from build123d import *

# Parameters (mm, degrees)
BOSS_EXTRUDE1_DEPTH = 2.25
BOSS_EXTRUDE2_DEPTH = 2
CHAMFER1_SIZE       = 2
SKETCH2_R           = 2.1
CUT_EXTRUDE3_DEPTH  = 4.25
BOSS_EXTRUDE3_REACH = 165.691
SKETCH4_W           = 30.977136558
SKETCH4_H           = 2.25


with BuildPart() as part:
    # Sketch1 → Boss-Extrude1 (new body)
    with BuildSketch(Plane(origin=(0, 30, 0), x_dir=(1, 0, 0), z_dir=(0, 1, 0))):
        with BuildLine():
            Line((16.150801753, 24.75), (-16.150801753, 24.75))
            ThreePointArc((-16.150801753, 24.75), (-28.096079542, 23.126243037), (-39.174486808, 18.372808426))
            Line((-39.174486808, 18.372808426), (-74.75, -2.97249949))
            Line((-74.75, -2.97249949), (-74.75, -31.794317372))
            add(Edge.make_bspline(
                [(-74.75, -31.794317372), (-74.75, -34.854957393), (-74.617964132, -37.896617098), (-74.092634279, -43.942380332), (-73.699378084, -46.946489294), (-72.640258958, -52.915519667), (-71.97459072, -55.880469065), (-70.750169489, -60.295417047), (-70.303298869, -61.763844969), (-69.338133577, -64.660739638), (-68.819099262, -66.092346674), (-67.147343369, -70.334199296), (-65.881052999, -73.091977263), (-63.717003155, -77.10639512), (-62.951317542, -78.424051782), (-61.728649984, -80.366285253), (-61.307989229, -81.009022825), (-60.443810311, -82.277119387), (-60.001044485, -82.901462706), (-57.731833326, -85.972836279), (-55.741550679, -88.270936188), (-52.431333352, -91.422844474), (-51.271504838, -92.425348837), (-48.832250491, -94.308303199), (-47.564474204, -95.179986516), (-46.242530751, -95.973152587)],
                knots=[0, 0, 0, 0, 0.125, 0.125, 0.25, 0.25, 0.375, 0.375, 0.4375, 0.4375, 0.5, 0.5, 0.625, 0.625, 0.6875, 0.6875, 0.71875, 0.71875, 0.75, 0.75, 0.875, 0.875, 0.9375, 0.9375, 1, 1, 1, 1], degree=3))
            Line((-46.242530751, -95.973152587), (-31.73109903, -104.68001162))
            add(Edge.make_bspline(
                [(-31.73109903, -104.68001162), (-29.275377335, -106.153444637), (-26.68234242, -107.275661914), (-22.580548307, -108.4161221), (-21.170611667, -108.705239228), (-18.343968581, -109.085294073), (-16.920969223, -109.178932188), (-15.488568279, -109.178932188)],
                knots=[0, 0, 0, 0, 0.5, 0.5, 0.75, 0.75, 1, 1, 1, 1], degree=3))
            Line((-15.488568279, -109.178932188), (15.488568279, -109.178932188))
            add(Edge.make_bspline(
                [(15.488568279, -109.178932188), (18.352407294, -109.178932188), (21.153292414, -108.807120107), (25.257313775, -107.674700988), (26.615074004, -107.197210462), (29.234437058, -106.068808934), (30.502825354, -105.416975826), (31.73109903, -104.68001162)],
                knots=[0, 0, 0, 0, 0.5, 0.5, 0.75, 0.75, 1, 1, 1, 1], degree=3))
            Line((31.73109903, -104.68001162), (46.242530751, -95.973152587))
            add(Edge.make_bspline(
                [(46.242530751, -95.973152587), (47.567869145, -95.177949551), (48.829466075, -94.309558847), (51.243712939, -92.447684976), (52.396262721, -91.454086815), (54.604509349, -89.355684378), (55.660153085, -88.25081912), (57.177112794, -86.517159458), (57.67228307, -85.925631056), (58.63283622, -84.728723238), (59.099288908, -84.122193289), (61.366991068, -81.05182626), (62.976708922, -78.476094674), (65.141118903, -74.466347585), (65.820469131, -73.105158474), (67.100436526, -70.336783684), (67.701854467, -68.927501042), (69.388296968, -64.647487304), (70.343996758, -61.758169069), (71.964810988, -55.917525955), (72.629539561, -52.966118736), (73.690525283, -47.006016439), (74.086644723, -43.997291976), (74.484256509, -39.442260691), (74.583986383, -37.915017565), (74.716839481, -34.856005184), (74.75, -33.325606239), (74.75, -31.794317372)],
                knots=[0, 0, 0, 0, 0.0625, 0.0625, 0.125, 0.125, 0.1875, 0.1875, 0.21875, 0.21875, 0.25, 0.25, 0.375, 0.375, 0.4375, 0.4375, 0.5, 0.5, 0.625, 0.625, 0.75, 0.75, 0.875, 0.875, 0.9375, 0.9375, 1, 1, 1, 1], degree=3))
            Line((74.75, -31.794317372), (74.75, -2.97249949))
            Line((74.75, -2.97249949), (39.174486808, 18.372808426))
            ThreePointArc((39.174486808, 18.372808426), (28.096079542, 23.126243037), (16.150801753, 24.75))
        make_face()
    extrude(amount=-BOSS_EXTRUDE1_DEPTH)

    # Sketch3 → Boss-Extrude2 (add)
    with BuildSketch(Plane(origin=(0, 30, 0), x_dir=(1, 0, 0), z_dir=(0, 1, 0))):
        with BuildLine():
            Line((16.150801753, 30), (-16.150801753, 30))
            ThreePointArc((-16.150801753, 30), (-29.497480847, 28.185746411), (-41.875589524, 22.874646286))
            Line((-41.875589524, 22.874646286), (-80, 0))
            Line((-80, 0), (-80, -31.794317372))
            add(Edge.make_bspline(
                [(-80, -31.794317372), (-80, -84.256429884), (-48.190171878, -103.342326757)],
                knots=[1.570796327, 1.570796327, 1.570796327, 2.769244761, 2.769244761, 2.769244761], degree=2, weights=[1, 0.825773406, 1]))
            Line((-48.190171878, -103.342326757), (-34.658026356, -111.46161407))
            add(Edge.make_bspline(
                [(-34.658026356, -111.46161407), (-26.260716473, -116.5), (-16.467854478, -116.5)],
                knots=[6.093295641, 6.093295641, 6.093295641, 6.473074974, 6.473074974, 6.473074974], degree=2, weights=[1, 0.982025067, 1]))
            Line((-16.467854478, -116.5), (16.467854478, -116.5))
            add(Edge.make_bspline(
                [(16.467854478, -116.5), (26.260716473, -116.5), (34.658026356, -111.46161407)],
                knots=[6.093295641, 6.093295641, 6.093295641, 6.473074974, 6.473074974, 6.473074974], degree=2, weights=[1, 0.982025067, 1]))
            Line((34.658026356, -111.46161407), (48.190171878, -103.342326757))
            add(Edge.make_bspline(
                [(48.190171878, -103.342326757), (80, -84.256429884), (80, -31.794317372)],
                knots=[0.372347892, 0.372347892, 0.372347892, 1.570796327, 1.570796327, 1.570796327], degree=2, weights=[1, 0.825773406, 1]))
            Line((80, -31.794317372), (80, 0))
            Line((80, 0), (41.875589524, 22.874646286))
            ThreePointArc((41.875589524, 22.874646286), (29.497480847, 28.185746411), (16.150801753, 30))
        make_face()
    extrude(amount=BOSS_EXTRUDE2_DEPTH)

    # Chamfer1
    chamfer1_edges = [part.edges().sort_by_distance(p)[0] for p in [
        (60.937794762, 32, -11.437323143),
        (80, 32, 15.897158686),
        (71.288670322, 32, 75.11613473),
        (41.424099117, 32, 107.401970414),
        (25.908664389, 32, 115.22898027),
        (0, 32, 116.5),
        (-25.908664389, 32, 115.22898027),
        (-41.424099117, 32, 107.401970414),
        (-71.288670322, 32, 75.11613473),
        (-80, 32, 15.897158686),
        (-60.937794762, 32, -11.437323143),
        (-29.497480847, 32, -28.185746411),
        (0, 32, -30),
        (29.497480847, 32, -28.185746411),
    ]]
    chamfer(chamfer1_edges, length=CHAMFER1_SIZE - 0.0001)  # a hair under: the kernel refuses the full size

    # Sketch2 → Cut-Extrude3 (cut)
    with BuildSketch(Plane(origin=(0, 32, 0), x_dir=(1, 0, 0), z_dir=(0, 1, 0))):
        with Locations(Location((66.361535838, -7.721967193, 0), (0, 0, 270))):
            Circle(SKETCH2_R)
        with Locations(Location((-66.361535838, -7.721967193, 0), (0, 0, 270))):
            Circle(SKETCH2_R)
    extrude(amount=-CUT_EXTRUDE3_DEPTH, mode=Mode.SUBTRACT)

    # Boss-Extrude3: up to this plane
    boss_extrude3_end = Plane(origin=(0, 26.464466094, 112.964466094), z_dir=(0, -0.7071067811865458, -0.7071067811865493))
    # Sketch4 → Boss-Extrude3 (add, up to the surface)
    with BuildSketch(Plane.XY.offset(109.178932188), mode=Mode.PRIVATE) as boss_extrude3_sk1:
        with Locations((0, 28.875)):
            Rectangle(SKETCH4_W, SKETCH4_H)
    boss_extrude3_tool1 = split(extrude(boss_extrude3_sk1.sketch, amount=BOSS_EXTRUDE3_REACH, mode=Mode.PRIVATE), bisect_by=boss_extrude3_end, keep=Keep.BOTH, mode=Mode.PRIVATE)
    add(boss_extrude3_tool1.solids().sort_by_distance((0, 28.875, 109.178932))[0])


solid = part.part
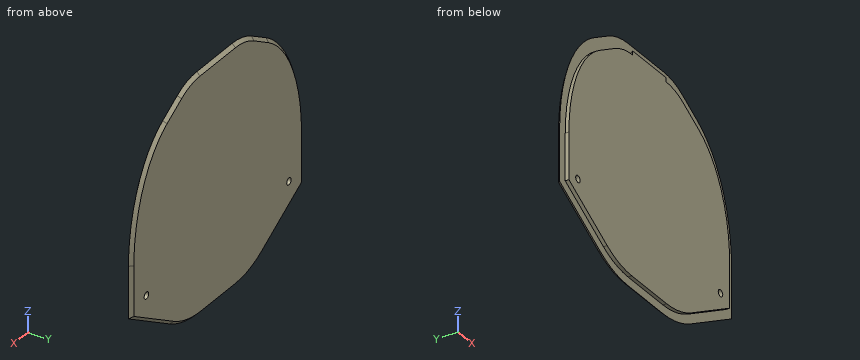
Geometry: final body of the model. Coordinates: model frame, mm. Give positions to 0.01 mm unless a question says otherwise; leave off trailing zeros. Return JSON: item names as keys, results as strings. Group by question number.
1) Line query: line 1 (X direction, y = 29.3, z = 6.5); line 2 (X direction, y = 29, z = 33.5); line 3 (Z direction, x = 68, y = 29.45). Output: solid intervals per line, ascending.
2) Section C-C on y = 31.25. State how many separate pieces and enclosed holes the cut face has, plus the area to 3 significant figures.
3) First-contact query: P1, Ø0.7, axis at x = 5, y = 28.5, coming from the -Z side; P2, Ø0.7, axis at y = 29, z = 110, coming from the -X side; P3, Ø1.8, axis at y = 28.5, z = 11, coming from the -X side. Flat tips, straight axial feed; report the tip coordinate or a pass-through.
Filled in:
{
 "1": {"line 1": "x = -74.75 to -68.07, -64.65 to 64.65, 68.07 to 74.75", "line 2": "x = -74.74 to 74.74", "line 3": "z = -1.08 to 6.41, 9.04 to 68.16"},
 "2": {"separate pieces": "1", "enclosed holes": "2", "area": "18,900 mm^2"},
 "3": {"P1": "stops at z = -24.75", "P2": "stops at x = -15.49", "P3": "stops at x = -74.75"}
}
